The listing builds one solid part. Answer for the finished solid, in the listing's coordinates (mm). Face numbers are marked on the shaded views. A direction names the side the tool comes from. Coordinates: 2 decimals unless noted, no trailing zeros. Order: outer loops, then holes, each group sorted by start corner. A loop starts at its lowest first (then second) coordinate and runs counter-clockwise, first axis right, second up. Notation, with made-up numbers: (36.5, -39.5) -> (82.5, -39.5) arc R33 cw to (82.5, -3.5) -> close; hole circle Ø10 at (-2, 7). An arc over 180 degrees is marked (long way). Write each question's results on one line, items separated by ' | '. Start each with the question number.
(1) A tool of negligible diameter and unlimited length cuts with its end or side. For the marked faces 4, 5 and 6, from which of +Z, -Z, +X, -X, +Y, -Y can it reach the whole face along a straight path? Write none if from no direction.
(2) Straight lines are drawn through the part: L1, parallel to X at y = 43.5, z = -0.5; L2, parallel to Y at x = -84, z = 21; L3, parallel to Y at x = 82, z = -32.5. For each, find the intervals that lie inside material, in ascending order.
(3) The part is cut by section A-A, the plane x = -41.5. Give the vertices of the cut face in (y, z), then the cut area to 3 significant figures.
(4) The part is cut by section D-D, the plane x = 36.5. Give the vertices of the cut face in (y, z).
(5) Determine the mould class of the marked faces 1, 2 and 3 for opening direction X: +X half, -X half, draft (parallel to the pull), parting line (faces both ways), or undercut.
(6) The part is cut by section B-B, the plane y = 48. Give the vertices of the cut face in (x, z), then the cut area to 3 significant figures.
(7) The part is cut by section C-C, the plane z = 1. Give the vertices of the cut face in (x, y).
(8) Given pin 1 (9 mm diameter, centred on x = 38, y = 37.5, fed in from +Z); pin 2 (7.5 mm diameter, centred on y = 5.5, z = 1.5, fed in from -X); pin 3 (8 mm diameter, centred on x = -110, z = -17, fed in from -Y), each flat-ended and moving along its own axis, determine where each tip first touches the part or whether it passes through.
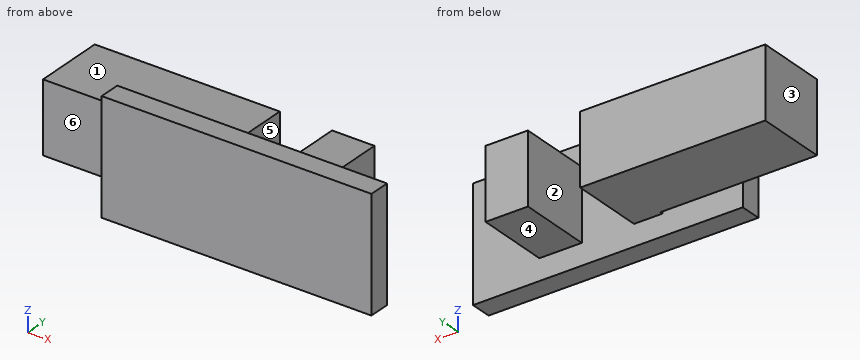
```python
from build123d import *

# Parameters (mm, degrees)
SKETCH1_W           = 191
SKETCH1_H           = 80
BOSS_EXTRUDE1_DEPTH = 15
SKETCH2_W           = 20
SKETCH2_H           = 50
SKETCH2_W_2         = 30
BOSS_EXTRUDE2_DEPTH = 52
SKETCH3_W           = 50
SKETCH3_H           = 50
BOSS_EXTRUDE3_DEPTH = 111


with BuildPart() as part:
    # Sketch1 → Boss-Extrude1 (new body)
    with BuildSketch(Plane(origin=(0, 0, 0), x_dir=(1, 0, 0), z_dir=(0, 1, 0))):
        Rectangle(SKETCH1_W, SKETCH1_H)
    extrude(amount=BOSS_EXTRUDE1_DEPTH)

    # Sketch2 → Boss-Extrude2 (add)
    with BuildSketch(Plane(origin=(0, 15, 0), x_dir=(1, 0, 0), z_dir=(0, 1, 0))):
        with Locations((-28.5, 0)):
            Rectangle(SKETCH2_W, SKETCH2_H)
        with Locations((33.5, 0)):
            Rectangle(SKETCH2_W_2, SKETCH2_H)
    extrude(amount=BOSS_EXTRUDE2_DEPTH)

    # Sketch3 → Boss-Extrude3 (add)
    with BuildSketch(Plane(origin=(-38.5, 0, 0), x_dir=(0, 0, -1), z_dir=(1, 0, 0))):
        with Locations((0, 42)):
            Rectangle(SKETCH3_W, SKETCH3_H)
    extrude(amount=-BOSS_EXTRUDE3_DEPTH)


solid = part.part
```
Established:
1) face 4: -Z, +X, -X, +Y | face 5: +Z, -Z, +Y | face 6: +Z, -Z, -X
2) L1: x = -149.5 to -18.5, 18.5 to 48.5 | L2: y = 0 to 15, 17 to 67 | L3: y = 0 to 15
3) outline: (0, -40) -> (15, -40) -> (15, 40) -> (0, 40) -> close; (17, -25) -> (67, -25) -> (67, 25) -> (17, 25) -> close | area: 3,700 mm^2
4) outline: (0, -40) -> (15, -40) -> (15, -25) -> (67, -25) -> (67, 25) -> (15, 25) -> (15, 40) -> (0, 40) -> close
5) face 1: draft | face 2: undercut | face 3: -X half
6) outline: (-149.5, -25) -> (-18.5, -25) -> (-18.5, 25) -> (-149.5, 25) -> close; (18.5, -25) -> (48.5, -25) -> (48.5, 25) -> (18.5, 25) -> close | area: 8,050 mm^2
7) outline: (-149.5, 17) -> (-38.5, 17) -> (-38.5, 15) -> (-95.5, 15) -> (-95.5, 0) -> (95.5, 0) -> (95.5, 15) -> (48.5, 15) -> (48.5, 67) -> (18.5, 67) -> (18.5, 15) -> (-18.5, 15) -> (-18.5, 67) -> (-149.5, 67) -> close
8) pin 1: stops at z = 25 | pin 2: stops at x = -95.5 | pin 3: stops at y = 17
